The listing builds one solid part. Answer for the finished solid, in the listing's coordinates (mm). Round coordinates to 2 decimals unless told otherwise and drop trailing zeros. Write each loop counter-clockwise with the first axis right and the second up, starting at its lowest first coordinate (ties: lowest second). Pieces come first, ordered by that corner, then holes. Notation, with made-up numbers: (-7.5, 54) - (-2.5, 54) arc R17 cw to (-2.5, 72) - close; hole circle Ø4 at (1, -40). An arc over 180 degrees is marked (long way). Answer in a Markdown table with one row per item.
from build123d import *

# Parameters (mm, degrees)
SKETCH2_W           = 326
SKETCH2_H           = 103
BOSS_EXTRUDE1_DEPTH = 3
CUT_EXTRUDE1_START  = -3
SKETCH3_R           = 10.2
CUT_EXTRUDE1_DEPTH  = 3


with BuildPart() as part:
    # Sketch2 → Boss-Extrude1 (new body)
    with BuildSketch(Plane(origin=(0, 0, 0), x_dir=(1, 0, 0), z_dir=(0, 1, 0))):
        Rectangle(SKETCH2_W, SKETCH2_H)
    extrude(amount=BOSS_EXTRUDE1_DEPTH)

    # Sketch3 → Cut-Extrude1 (cut)
    with BuildSketch(Plane(origin=(0, 3, 0), x_dir=(1, 0, 0), z_dir=(0, 1, 0)).offset(CUT_EXTRUDE1_START)):
        with Locations(Location((-88, 8.5, 0), (0, 0, 270))):
            Circle(SKETCH3_R)
        with Locations(Location((88, 8.5, 0), (0, 0, 270))):
            Circle(SKETCH3_R)
        with Locations(Location((-40.4, -18.7, 0), (0, 0, 270))):
            Circle(SKETCH3_R)
        with Locations(Location((0, -18.7, 0), (0, 0, 270))):
            Circle(SKETCH3_R)
        with Locations(Location((40.4, -18.7, 0), (0, 0, 270))):
            Circle(SKETCH3_R)
    extrude(amount=CUT_EXTRUDE1_DEPTH, mode=Mode.SUBTRACT)


solid = part.part
(1) Section A-A (x = 40.4) is taken. Give the vertices of the cut face in (y, z), and give its area (3 significant figures).
Checked values:
| item | result |
|---|---|
| outline | (0, -51.5) - (3, -51.5) - (3, 8.5) - (0, 8.5) - close; (0, 28.9) - (3, 28.9) - (3, 51.5) - (0, 51.5) - close |
| area | 248 mm2 |
(2) For a pull along Z with two mould halves and no side action, classify faces 1 (the cylindrical face through (30.443, 1.479, 16.489)), 2 (the flat face through (-2, 0, -1)), 3 (the cylindrical face through (-94.2, 1.5, -16.6)) as pulls with the +Z half, pulls with the -Z half, needs draft (parallel to the pull), parting line crosses it, or undercut.
Checked values:
| item | result |
|---|---|
| face 1 | undercut |
| face 2 | needs draft |
| face 3 | undercut |
(3) Section C-C (y = 2.1) is taken. Give the vertices of the cut face in (x, z).
Checked values:
| item | result |
|---|---|
| outline | (-163, -51.5) - (163, -51.5) - (163, 51.5) - (-163, 51.5) - close; hole circle Ø20.4 at (-88, -8.5); hole circle Ø20.4 at (-40.4, 18.7); hole circle Ø20.4 at (0, 18.7); hole circle Ø20.4 at (40.4, 18.7); hole circle Ø20.4 at (88, -8.5) |
(4) Section B-B (z = 18.7) is taken. Give the vertices of the cut face in (x, y), and give its area (3 significant figures).
Checked values:
| item | result |
|---|---|
| outline | (-163, 0) - (-50.6, 0) - (-50.6, 3) - (-163, 3) - close; (-30.2, 0) - (-10.2, 0) - (-10.2, 3) - (-30.2, 3) - close; (10.2, 0) - (30.2, 0) - (30.2, 3) - (10.2, 3) - close; (50.6, 0) - (163, 0) - (163, 3) - (50.6, 3) - close |
| area | 794 mm2 |
(5) Section D-D (z = -8.5) is taken. Give the vertices of the cut face in (x, y).
Checked values:
| item | result |
|---|---|
| outline | (-163, 0) - (-98.2, 0) - (-98.2, 3) - (-163, 3) - close; (-77.8, 0) - (77.8, 0) - (77.8, 3) - (-77.8, 3) - close; (98.2, 0) - (163, 0) - (163, 3) - (98.2, 3) - close |
(6) Find the intervals of material crossed by line 1 (X direction, y = 2.05, z = 18.7); line 2 (X direction, y = 1.85, z = -8.5); line 3 (X direction, y = 2.7, z = 13), in increasing order.
Checked values:
| item | result |
|---|---|
| line 1 | x = -163 to -50.6, -30.2 to -10.2, 10.2 to 30.2, 50.6 to 163 |
| line 2 | x = -163 to -98.2, -77.8 to 77.8, 98.2 to 163 |
| line 3 | x = -163 to -48.86, -31.94 to -8.46, 8.46 to 31.94, 48.86 to 163 |
